Job drawing, mm, ordinate dimensions from the low corner. One solid piece. Give positions to 0.01 mm unless a question says otherwise; leave off trailing zeros. Loops run counter-clockwise (first coordinate to the right, second up) from the corner with the lowest first, then second, coordinate; pieces in that order, holes last. Notation, with made-up numbers: M 36,12.25 L 94,12.25 A20 cw 94,28.25 Z; hole C 25.5,39 d10. An arc over 180 degrees is marked long. One line per question, with ' | ' between items.
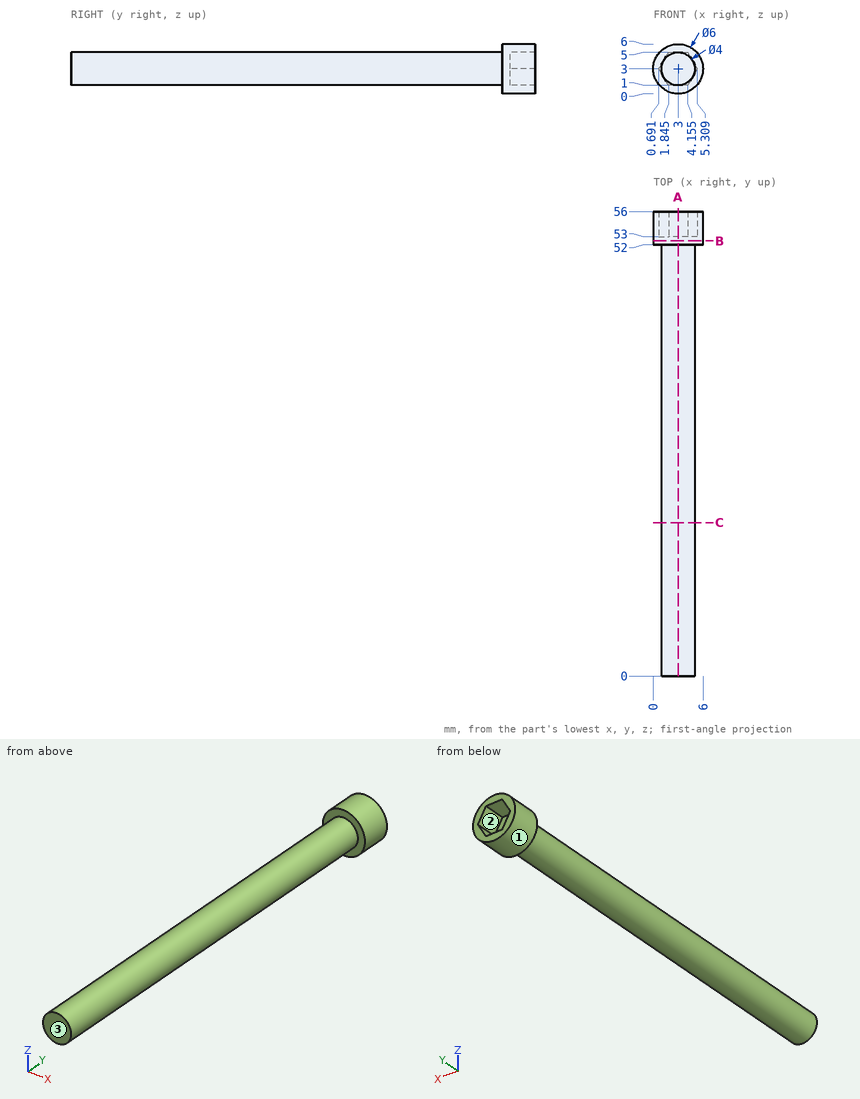
Item 1: Drop flat-ended pins along their axis: P1, Ø1.8, axis at x = 2.5, y = 55, coming from the -Z side; P2, Ø1.2, axis at x = 3.5, z = 2.5, coming from the +Y side; P3, Ø2, axis at x = 2.5, y = 22.5, coming from the +Z side. Give the stop position or say it passes through.
Conclusion:
P1: z = 0 | P2: y = 53 | P3: z = 5
Item 2: Drill centre lines: line 1 along Y through (x, z) = (3.1, 0.65); line 2 along Y through (x, z) = (1.65, 1.95); line 3 along X through (y, z) = (46, 2.85) (1 decimal). Where is each one in solid material? Low to high. Write a range as [from, to].
Conclusion:
line 1: [52, 56] | line 2: [0, 53] | line 3: [1, 5]
Item 3: Saw through at B-B on y = 52.5. Give the cut face in (x, z), and give its area (3 significant figures).
Conclusion:
outline: C 3,3 d6 | area: 28.3 mm²
Item 4: Saw through at A-A on x = 3. Give the cut face in (y, z), and give its area (3 significant figures).
Conclusion:
outline: M 0,1 L 52,1 L 52,0 L 56,0 L 56,1 L 53,1 L 53,5 L 56,5 L 56,6 L 52,6 L 52,5 L 0,5 Z | area: 220 mm²
Item 5: Saw through at C-C on y = 18.5. Give the cut face in (x, z), and give its area (3 significant figures).
Conclusion:
outline: C 3,3 d4 | area: 12.6 mm²
Item 6: Mould opens along X. For the marked faces 1, 2 and 3 say: pulls with the +X half, pulls with the -X half, needs draft (parallel to the pull), parting line crosses it, or undercut.
Conclusion:
face 1: parting line crosses it | face 2: undercut | face 3: needs draft
